```python
from build123d import *

# Parameters (mm, degrees)
F1_DEPTH = 12.7
F2_DEPTH = 27.94
F3_W     = 152.38668
F3_H     = 38.1
F4_DEPTH = 12.7


with BuildPart() as f1:
    # F0 (on Front) → F1 (new body)
    with BuildSketch(Plane.XZ):
        Polygon((368.3, 19.05), (-368.3, 19.05), (-368.3, -6.35), (-228.6, -6.35), (-228.6, -19.05), (228.6, -19.05), (228.6, -6.35), (368.3, -6.35), align=None)
        Polygon((-368.3, 19.05), (-381, 19.05), (-381, -19.05), (-228.6, -19.05), (-228.6, -6.35), (-368.3, -6.35), align=None)
        Polygon((381, 19.05), (368.3, 19.05), (368.3, -6.35), (228.6, -6.35), (228.6, -19.05), (381, -19.05), align=None)
    extrude(amount=-F1_DEPTH)

    # F0 (on Front) → F2 (join)
    with BuildSketch(Plane.XZ):
        Polygon((-368.3, 19.05), (-381, 19.05), (-381, -19.05), (-228.6, -19.05), (-228.6, -6.35), (-368.3, -6.35), align=None)
        Polygon((381, 19.05), (368.3, 19.05), (368.3, -6.35), (228.6, -6.35), (228.6, -19.05), (381, -19.05), align=None)
    extrude(amount=F2_DEPTH)

    # F3 (on face) → F4 (join)
    with BuildSketch(Plane.XZ.offset(27.94)):
        Polygon((-368.3, 19.05), (-381, 19.05), (-381, -19.05), (-228.6, -19.05), (-228.6, 19.05), align=None)
        with Locations((305.05722, 0)):
            Rectangle(F3_W, F3_H)
    extrude(amount=F4_DEPTH)


solid = f1.part
```
Source: CAD feature listing. Evaluate the final solid. Frame: model axes, mm. A direction names the side the tool comes from. Round coordinates to 2 decimals unless told otherwise and drop trailing zeros. Loops run counter-clockwise (first coordinate to the right, second up) from the corner with the lowest first, then second, coordinate; pieces in that order, holes last. Notation, with made-up numbers: M -5,-11 L 45,-11 A13 ccw 45,12 Z; hole C 13.5,60.25 d8. An arc over 180 degrees is marked long. Use a Markdown table: item, result. Add a question column.
1. Contact query for flat-ended pins moving along their axis: pin 1 (10 mm diameter, centred on x = -71, y = -9, fed in from +Z); pin 2 (14 mm diameter, centred on x = -306, y = -17, fed in from +Z); pin 3 (2 mm diameter, centred on x = -125.5, z = -9, fed in from -Y); pin 4 (20.5 mm diameter, centred on y = -10, z = 0.5, fed in from +X). Output: stop coordinate, or through.
2. Cut plane B-B, the plane z = 7.5. Output: boundary loops of the cut face in (x, y), and give its area (3 significant figures).
3. Pull-direction query (X, two-part tool) for faces 4 (the flat face through (228.6, -14, -13)), 5 (the flat face through (-381, -14, 0)), 6 (the flat face through (381, -8, 0)); classes: +X half, -X half, draft (parallel to the pull), parting line (faces both ways), or undercut.
4. Cut plane C-C, the plane x = -327. Output: boundary loops of the cut face in (y, z).
5. Set-up query: faces 1 (the flat face through (368.3, -14, 7)), 2 (the flat face through (-228.6, -25, -9)), 3 (the flat face through (30, 6, 19.05)). Return all of +Z, -Z, +X, -X, +Y, -Y with unobstructed straight access to the full face (end or side cutting, diameter ignored); none if empty.
6. Cut plane D-D, the plane x = 50. Output: boundary loops of the cut face in (y, z).
7. Ray query, line 1 along X through (y, z) = (-24.5, 7.5); line 2 along X through (y, z) = (-29, 5); line 3 along Y through (x, z) = (252, 17.5). Return the intervals inside material, ascending. Write a range as [from, to].
8. Cut plane A-A, the plane y = -20. Output: boundary loops of the cut face in (x, z), and give its area (3 significant figures).
Solution:
| question | item | result |
|---|---|---|
| 1 | pin 1 | passes through |
| 1 | pin 2 | stops at z = -6.35 |
| 1 | pin 3 | stops at y = 0 |
| 1 | pin 4 | stops at x = 381 |
| 2 | outline | M -381,-40.64 L -228.6,-40.64 L -228.6,-27.94 L -368.3,-27.94 L -368.3,0 L 368.3,0 L 368.3,-27.94 L 228.86,-27.94 L 228.86,-40.64 L 381.25,-40.64 L 381.25,-27.94 L 381,-27.94 L 381,12.7 L -381,12.7 Z |
| 2 | area | 14,300 mm2 |
| 3 | face 4 | undercut |
| 3 | face 5 | -X half |
| 3 | face 6 | +X half |
| 4 | outline | M -40.64,-19.05 L 12.7,-19.05 L 12.7,19.05 L 0,19.05 L 0,-6.35 L -27.94,-6.35 L -27.94,19.05 L -40.64,19.05 Z |
| 5 | face 1 | +Z |
| 5 | face 2 | +Z, -Z, -Y |
| 5 | face 3 | +Z, +X, -X, +Y, -Y |
| 6 | outline | M 0,-19.05 L 12.7,-19.05 L 12.7,19.05 L 0,19.05 Z |
| 7 | line 1 | x = [-381, -368.3], [368.3, 381] |
| 7 | line 2 | x = [-381, -228.6], [228.86, 381.25] |
| 7 | line 3 | y = [-40.64, -27.94], [0, 12.7] |
| 8 | outline | M -381,-19.05 L -228.6,-19.05 L -228.6,-6.35 L -368.3,-6.35 L -368.3,19.05 L -381,19.05 Z; M 228.6,-19.05 L 381,-19.05 L 381,19.05 L 368.3,19.05 L 368.3,-6.35 L 228.6,-6.35 Z |
| 8 | area | 4,520 mm2 |
